from build123d import *

# Parameters (mm, degrees)
EXTRUDE_3_DEPTH     = 3
EXTRUDE_START       = 0.8
EXTRUDE_4_DEPTH     = 0.8
SKETCH_4_W          = 3
SKETCH_4_H          = 15.25
CUT_EXTRUDE_1_DEPTH = 4
SKETCH_5_W          = 10.25
SKETCH_5_H          = 3.645381057
CUT_EXTRUDE_2_DEPTH = 3
SKETCH_6_W          = 2.899645865
SKETCH_6_H          = 1.169365381
SKETCH_6_H_2        = 1.169365382
CUT_EXTRUDE_3_DEPTH = 3.2
CUT_EXTRUDE_5_REACH = 30.478
SKETCH_7_W          = 2.785841709
SKETCH_7_H          = 1.637134251
SKETCH_7_W_2        = 2.809808384
SKETCH_7_H_2        = 1.583820861
CUT_EXTRUDE_6_REACH = 30.478
SKETCH_8_W          = 2.793582113
SKETCH_8_H          = 1.569963741
SKETCH_8_W_2        = 2.785085694
SKETCH_8_H_2        = 1.60265935


with BuildPart() as part:
    # 草图1 → 凸台-拉伸3 (new body)
    with BuildSketch(Plane(origin=(0, 0, 0), x_dir=(1, 0, 0), z_dir=(0, 1, 0))):
        with BuildLine():
            Line((-16, 10.5), (16, 10.5))
            ThreePointArc((16, 10.5), (18.121320344, 9.621320344), (19, 7.5))
            Line((19, 7.5), (19, -7.5))
            ThreePointArc((19, -7.5), (18.121320344, -9.621320344), (16, -10.5))
            Line((16, -10.5), (-16, -10.5))
            ThreePointArc((-16, -10.5), (-18.121320344, -9.621320344), (-19, -7.5))
            Line((-19, -7.5), (-19, 7.5))
            ThreePointArc((-19, 7.5), (-18.121320344, 9.621320344), (-16, 10.5))
        make_face()
        with BuildLine():
            Line((-16, 9), (16, 9))
            ThreePointArc((16, 9), (17.060660172, 8.560660172), (17.5, 7.5))
            Line((17.5, 7.5), (17.5, -7.5))
            ThreePointArc((17.5, -7.5), (17.060660172, -8.560660172), (16, -9))
            Line((16, -9), (-16, -9))
            ThreePointArc((-16, -9), (-17.060660172, -8.560660172), (-17.5, -7.5))
            Line((-17.5, -7.5), (-17.5, 7.5))
            ThreePointArc((-17.5, 7.5), (-17.060660172, 8.560660172), (-16, 9))
        make_face(mode=Mode.SUBTRACT)
    extrude(amount=EXTRUDE_3_DEPTH)

    # 草图3 → 凸台-拉伸4 (add)
    with BuildSketch(Plane.XZ.offset(EXTRUDE_START)):
        with BuildLine():
            Line((-16, 10.5), (16, 10.5))
            ThreePointArc((16, 10.5), (18.121320344, 9.621320344), (19, 7.5))
            Line((19, 7.5), (19, -7.5))
            ThreePointArc((19, -7.5), (18.121320344, -9.621320344), (16, -10.5))
            Line((16, -10.5), (-16, -10.5))
            ThreePointArc((-16, -10.5), (-18.121320344, -9.621320344), (-19, -7.5))
            Line((-19, -7.5), (-19, 7.5))
            ThreePointArc((-19, 7.5), (-18.121320344, 9.621320344), (-16, 10.5))
        make_face()
    extrude(amount=-EXTRUDE_4_DEPTH)

    # 草图4 → 切除-拉伸1 (cut)
    with BuildSketch(Plane(origin=(0, 3, 0), x_dir=(1, 0, 0), z_dir=(0, 1, 0))):
        with Locations((-19, 0)):
            Rectangle(SKETCH_4_W, SKETCH_4_H)
    extrude(amount=-CUT_EXTRUDE_1_DEPTH, mode=Mode.SUBTRACT)

    # 草图5 → 切除-拉伸2 (cut)
    with BuildSketch(Plane(origin=(19, 0, 0), x_dir=(0, 0, -1), z_dir=(1, 0, 0))):
        with Locations((-0.144, 3.148589472)):
            Rectangle(SKETCH_5_W, SKETCH_5_H)
    extrude(amount=-CUT_EXTRUDE_2_DEPTH, mode=Mode.SUBTRACT)

    # 草图6 → 切除-拉伸3 (cut)
    with BuildSketch(Plane(origin=(0, 3, 0), x_dir=(1, 0, 0), z_dir=(0, 1, 0))):
        with Locations((9.842196581, -9.77321518)):
            Rectangle(SKETCH_6_W, SKETCH_6_H)
        with Locations((-9.847989742, -9.777101279)):
            Rectangle(SKETCH_6_W, SKETCH_6_H_2)
        with Locations((9.842196581, 9.77321518)):
            Rectangle(SKETCH_6_W, SKETCH_6_H)
        with Locations((-9.847989742, 9.777101279)):
            Rectangle(SKETCH_6_W, SKETCH_6_H_2)
    extrude(amount=-CUT_EXTRUDE_3_DEPTH, mode=Mode.SUBTRACT)

    # 切除-拉伸5: up to this face of the body (flat: up to its plane)
    cut_extrude_5_end = Plane(part.part.faces().sort_by_distance((9.84219658, 1.4, -10.357897871))[0])
    # 草图7 → 切除-拉伸5 (cut, up to the picked face)
    with BuildSketch(Plane(origin=(0, 0, -10.5), x_dir=(-1, 0, 0), z_dir=(0, 0, -1)), mode=Mode.PRIVATE) as cut_extrude_5_sk1:
        with Locations((9.877407398, 0.717488498)):
            Rectangle(SKETCH_7_W, SKETCH_7_H)
    cut_extrude_5_tool1 = split(extrude(cut_extrude_5_sk1.sketch, amount=-CUT_EXTRUDE_5_REACH, mode=Mode.PRIVATE), bisect_by=cut_extrude_5_end, keep=Keep.BOTH, mode=Mode.PRIVATE)
    # 草图7 → 切除-拉伸5 (cut, up to the picked face)
    with BuildSketch(Plane(origin=(0, 0, -10.5), x_dir=(-1, 0, 0), z_dir=(0, 0, -1)), mode=Mode.PRIVATE) as cut_extrude_5_sk2:
        with Locations((-9.836726154, 0.744145193)):
            Rectangle(SKETCH_7_W_2, SKETCH_7_H_2)
    cut_extrude_5_tool2 = split(extrude(cut_extrude_5_sk2.sketch, amount=-CUT_EXTRUDE_5_REACH, mode=Mode.PRIVATE), bisect_by=cut_extrude_5_end, keep=Keep.BOTH, mode=Mode.PRIVATE)
    add(cut_extrude_5_tool1.solids().sort_by(Axis((-9.877407, 0.717488, -10.5), (0, 0, 1)))[0], mode=Mode.SUBTRACT)
    add(cut_extrude_5_tool2.solids().sort_by(Axis((9.836726, 0.744145, -10.5), (0, 0, 1)))[0], mode=Mode.SUBTRACT)

    # 草图8 → 切除-拉伸6 (cut, up to next)
    with BuildSketch(Plane.XY.offset(10.5), mode=Mode.PRIVATE) as cut_extrude_6_sk1:
        with Locations((9.840094375, 0.730022081)):
            Rectangle(SKETCH_8_W, SKETCH_8_H)
    cut_extrude_6_tool1 = extrude(cut_extrude_6_sk1.sketch, amount=-CUT_EXTRUDE_6_REACH, mode=Mode.PRIVATE) & part.part
    # 草图8 → 切除-拉伸6 (cut, up to next)
    with BuildSketch(Plane.XY.offset(10.5), mode=Mode.PRIVATE) as cut_extrude_6_sk2:
        with Locations((-9.878038676, 0.698670325)):
            Rectangle(SKETCH_8_W_2, SKETCH_8_H_2)
    cut_extrude_6_tool2 = extrude(cut_extrude_6_sk2.sketch, amount=-CUT_EXTRUDE_6_REACH, mode=Mode.PRIVATE) & part.part
    add(cut_extrude_6_tool1.solids().sort_by_distance((9.840094, 0.730022, 10.5))[0], mode=Mode.SUBTRACT)
    add(cut_extrude_6_tool2.solids().sort_by_distance((-9.878039, 0.69867, 10.5))[0], mode=Mode.SUBTRACT)


solid = part.part
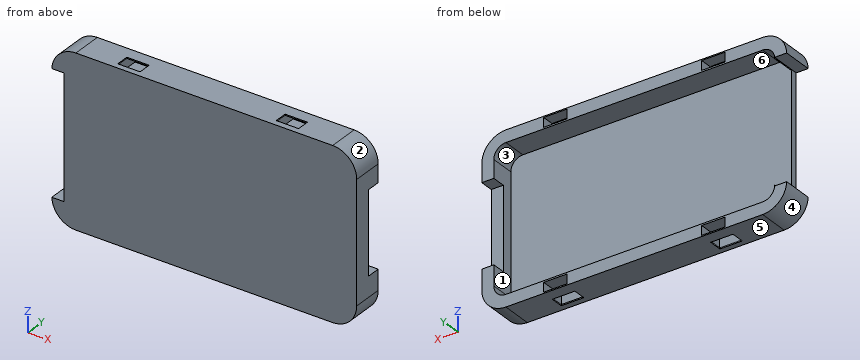
Verification items for the finished model (mm, model axes). Face numbers are marked on the shaded views. A direction names the side the tool comes from. Round coordinates to 2 decimals unless told otherwise and drop trailing zeros. Order: outer loops, then holes, each group sorted by start corner. A loop starts at its lowest first (then second) coordinate and runs counter-clockwise, first axis right, second up. Notation, with made-up numbers: (16.25, 6) -> (41.25, 6) arc R28 cw to (41.25, 29) -> close; hole circle Ø10 at (56.25, -35). An arc over 180 degrees is marked (long way). Put each result on its own line as item: value.
1) Set-up check for the marked faces 1, 2 and 3: record each of +Z, -Z, +X, -X, +Y, -Y from which the full face is reachable in a straight line by a thin tool's end or side.
Final values:
face 1: -X, +Y
face 2: +Z, +X, +Y, -Y
face 3: +Y
2) Section check B-B (z = 3.25). Record the cut outline in (x, y).
Final values:
outline: (-17.5, -0.8) -> (19, -0.8) -> (19, 1.33) -> (17.5, 1.33) -> (17.5, 0) -> (-17.5, 0) -> close
3) Section check D-D (z = -8.5). Record the cut outline in (x, y), then the cut area to 3 significant figures.
Final values:
outline: (-18.83, -0.8) -> (18.83, -0.8) -> (18.83, 3) -> (17.12, 3) -> (17.12, 0) -> (-17.12, 0) -> (-17.12, 3) -> (-18.83, 3) -> close
area: 40.4 mm^2
4) Section check C-C (z = 7). Record the cut outline in (x, y).
Final values:
outline: (-17.5, -0.8) -> (19, -0.8) -> (19, 3) -> (17.5, 3) -> (17.5, 0) -> (-17.5, 0) -> close
5) Mould release check, pull along X, two halves, no side actions. Record for the marked faces 4, 5 and 6: +X half, -X half, draft (parallel to the pull), parting line (faces both ways), or undercut.
Final values:
face 4: -X half
face 5: draft
face 6: undercut
6) Depth check by flat-ended pin: pin 1 (0.9 mm diameter, centred on y = 1, z = 10, fed in from +X); pin 2 (1.3 mm diameter, centred on y = 1, z = -9.5, fed in from -X); pin 3 (0.9 mm diameter, centred on x = -10, z = 9.5, fed in from +Y). Enter the tip coordinate at first touch or a pass-through.
Final values:
pin 1: stops at x = 18.19
pin 2: stops at x = -18.68
pin 3: stops at y = 3
7) Material ranges on line 1 (Z direction, x = 14, y = 1.3); line 2 (X direction, y = 1.35, z = -9.25); line 3 (Z direction, x = 10, y = 0.3), recorded low to high.
Final values:
line 1: z = -10.5 to -9, 9 to 10.5
line 2: x = -18.44 to -11.3, -8.4 to 8.39, 11.29 to 18.44
line 3: z = -9.19 to -9, 9 to 9.19
8) Section check A-A (x = -13). Record the cut outline in (y, z).
Final values:
outline: (-0.8, -10.5) -> (3, -10.5) -> (3, -9) -> (0, -9) -> (0, 9) -> (3, 9) -> (3, 10.5) -> (-0.8, 10.5) -> close
